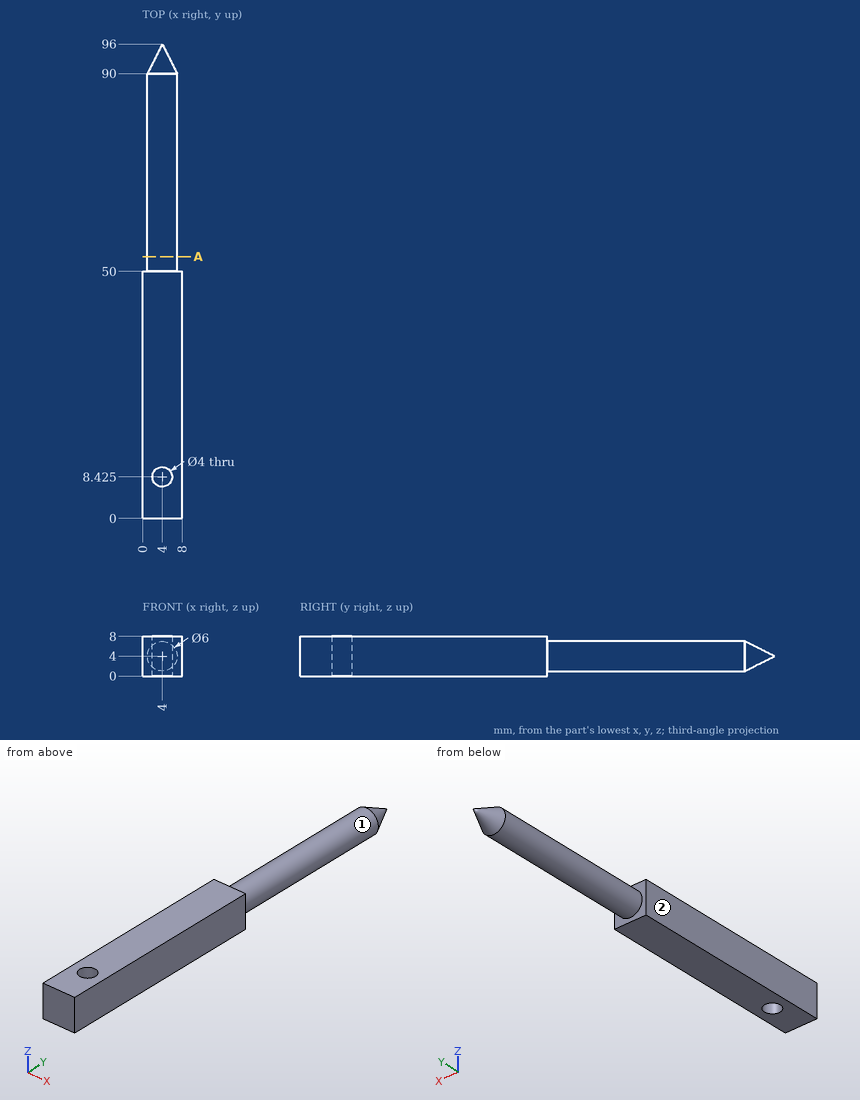
The drawing under review shows one solid part. Ordinate dimensions are in mm from its lowest x, y, z. A direction names the side the tool comes from. Give positions to 0.01 mm unless a question says otherwise; leave off trailing zeros. Loops run counter-clockwise (first coordinate to the right, second up) from the corner with the lowest first, then second, coordinate; pieces in that order, holes last. Notation, with made-up numbers: M -21,79 L -2,79 A29 cw -2,110 Z; hole C 1,-6.5 d7. An arc over 180 degrees is marked long. One line per question, with ' | ' between items. Start each with the question number.
1. Insertion check: P1, Ø1.5, axis at x = 6, y = 64, coming from the -Z side; P2, Ø2.5, axis at x = 2, z = 3, coming from the +Y side; P3, Ø4, axis at y = 73, z = 4.5, coming from the +X side. Each pin has a flat end and moves straight along its axis. Give the tip position at first contact, or say it passes through.
2. Add section A-A (y = 53). Write out the cut boundary in (x, z), plus the area to 3 significant figures.
3. To check wall thickness, follow L1, parallel to Y at x = 3.25, z = 6.75; L2, parallel to Y at x = 0.5, z = 6.5; L3, parallel to X at y = 75.5, z = 4.25. State the ranges of each line that lie inside material, in increasing order.
4. For the marked faces 1 and 2, list the 3-axis set-ups (+Z, -Z, +X, -X, +Y, -Y) from which the entire face can be reached by the end or side of a thin tool; tool diameter is ignored.
Worked out:
1) P1: stops at z = 1.27 | P2: stops at y = 94.03 | P3: stops at x = 7
2) outline: C 4,4 d6 | area: 28.3 mm²
3) L1: y = 0 to 6.57, 10.28 to 90.3 | L2: y = 0 to 50 | L3: x = 1.01 to 6.99
4) face 1: +Y | face 2: +Z, -Z, -X, +Y, -Y
